```python
from build123d import *

# Parameters (mm, degrees)
CONG_1_R    = 0.4
CONG_2_R    = 0.8
ESQUISSE2_R = 5.05
CONG_3_R    = 4


with BuildPart() as part:
    # Esquisse1 → Révolution1 (revolve)
    with BuildSketch(Plane.XY):
        Polygon((0, 64.88), (4.5, 64.88), (4.5, 63.147633926), (5.788540515, 63.147633926), (5.788540515, 64.5), (4.8, 64.5), (4.8, 64.7), (6.25, 64.7), (6.25, 64.88), (9.1, 64.88), (9.1, 0), (7, 0), (7, 0.18), (0, 0.18), align=None)
    revolve(axis=Axis((0, 0, 0), (0, 1, 0)))

    # Congé1
    cong_1_edges = [part.edges().sort_by_distance(p)[0] for p in [
        (-4.5, 64.88, 0),
    ]]
    fillet(cong_1_edges, radius=CONG_1_R)

    # Congé2
    cong_2_edges = [part.edges().sort_by_distance(p)[0] for p in [
        (-9.1, 0, 0),
        (-9.1, 64.88, 0),
    ]]
    fillet(cong_2_edges, radius=CONG_2_R)

    # Esquisse2 → Enlèvement de matière-Révolution1 (revolve, cut)
    with BuildSketch(Plane(origin=(0, 0, 0), x_dir=(0, 0, -1), z_dir=(1, 0, 0))):
        with Locations((14.05, 61.04)):
            Circle(ESQUISSE2_R)
    revolve(axis=Axis((0, 52.453065443, 0), (0, 1, 0)), mode=Mode.SUBTRACT)

    # Congé3
    cong_3_edges = [part.edges().sort_by_distance(p)[0] for p in [
        (6.434671709, 62.04, -6.434671709),
        (-6.434671709, 60.04, 6.434671709),
    ]]
    fillet(cong_3_edges, radius=CONG_3_R)


solid = part.part
```
Geometry check sheet. Reference: the model listing, model coordinates, mm. A direction names the side the tool comes from. Round coordinates to 2 decimals unless told otherwise and drop trailing zeros. Loops run counter-clockwise (first coordinate to the right, second up) from the corner with the lowest first, then second, coordinate; pieces in that order, holes last. Notation, with made-up numbers: (15.25, -15.75) -> (36.25, -15.75) arc R13 ccw to (36.25, 5.25) -> close; hole circle Ø1 at (-8.75, -16). An arc over 180 degrees is marked (long way). Use a Markdown table: item, result.
(1) Go/stop test with flat-tipped pins: P1, Ø7.5, axis at x = 0, z = 0, coming from the -Y side; P2, Ø4, axis at x = -6.5, y = 58, coming from the +Z side; P3, Ø4, axis at x = -2.5, y = 41.5, coming from the -Z side. Record where each tip stops, or that it passes through.
Calculated:
| item | result |
|---|---|
| P1 | y = 0.18 |
| P2 | z = 7.91 |
| P3 | z = -9.09 |
(2) Sectioned sample at A-A (y = 35). Enter the section's corners in (x, z), then the cut area to 3 significant figures.
Calculated:
| item | result |
|---|---|
| outline | circle Ø18.2 at (0, 0) |
| area | 260 mm² |
(3) Mould release check, pull along Z, two halves, no side actions. Record for faces 6 (the cylindrical face through (-1.973, 63.219, 8.884)), 7 (the flat face through (1, 64.5, -5)), 8 (the flat face through (0, 64.88, 0)): released by +Z, released by -Z, zero draft, split by the parting line, or undercut.
Calculated:
| item | result |
|---|---|
| face 6 | split by the parting line |
| face 7 | undercut |
| face 8 | zero draft |
(4) Set-up check for faces 1 (the flat face through (0, 0.18, 0)), 2 (the flat face through (-3, 64.88, -6)), 3 (the flat face through (-4, 0, 6)), 4 (the cylindrical face through (-0.59, 63.8, -4.46)), 5 (the cylindrical face through (-0.75, 63.83, -5.74)): record each of +Z, -Z, +X, -X, +Y, -Y from which the full face is reachable in a straight line by a thin tool's end or side.
Calculated:
| item | result |
|---|---|
| face 1 | -Y |
| face 2 | +Z, -Z, +X, -X, +Y |
| face 3 | +Z, -Z, +X, -X, -Y |
| face 4 | +Y |
| face 5 | none |
(5) Scan lines: probe 1 along X at (y, z) = (63.4, 0); probe 2 along Z at (x, y) = (0, 64.8). Record each from-to range of solid material in increasing order.
Calculated:
| item | result |
|---|---|
| probe 1 | -9.1 to -5.79, -4.5 to 4.5, 5.79 to 9.1 |
| probe 2 | -8.65 to -6.25, -4.34 to 4.34, 6.25 to 8.65 |
